Input: dimensioned drawing with shaded views. Units: mm. Origin: part minimum x, y, z. Round coordinates to 2 decimals unless told otherwise and drop trailing zeros. Order: outer loops, then holes, each group sorted by start corner. A loop starts at its lowest first (then second) coordinate and runs counter-clockwise, first axis right, second up. Notation, with made-up numbers: (66.5, 7) - (91.5, 7) arc R19 cw to (91.5, 17) - close; hole circle Ø7 at (86.5, -4). An arc over 180 degrees is marked (long way). Put each result on its own line as item: value. Start each with the question number.
(1) Section B-B (z = 10). Output: boundary loops of the cut face in (x, y), and give its area (3 significant figures).
(2) Section C-C (y = 56.5). Output: boundary loops of the cut face in (x, z), and give its area (3 significant figures).
(3) Material intervals for L1, parallel to Y at x = 21, z = 25; L2, parallel to Y at x = 24.5, z = 5.5 (1 decimal); L3, parallel to X at y = 62.5, z = 31.5, sorted ascending. Write a range as [from, to].
(4) Section D-D (y = 7.5). Output: boundary loops of the cut face in (x, z), and give its area (3 significant figures).
(5) Section A-A (x = 11.5). Output: boundary loops of the cut face in (y, z), and give its area (3 significant figures).
(6) Pin query (flat end, axial travel): P1, Ø5, axis at x = 27.5, y = 57.5, coming from the +Z side; P2, Ø5, axis at x = 12, z = 41.5, coming from the -Y side; P3, Ø10, axis at x = 24.5, y = 27.5, coming from the +Z side; P4, Ø2, axis at y = 11.5, z = 18, coming from the +X side. Return the tip coordinate at first contact, or that it passes through.
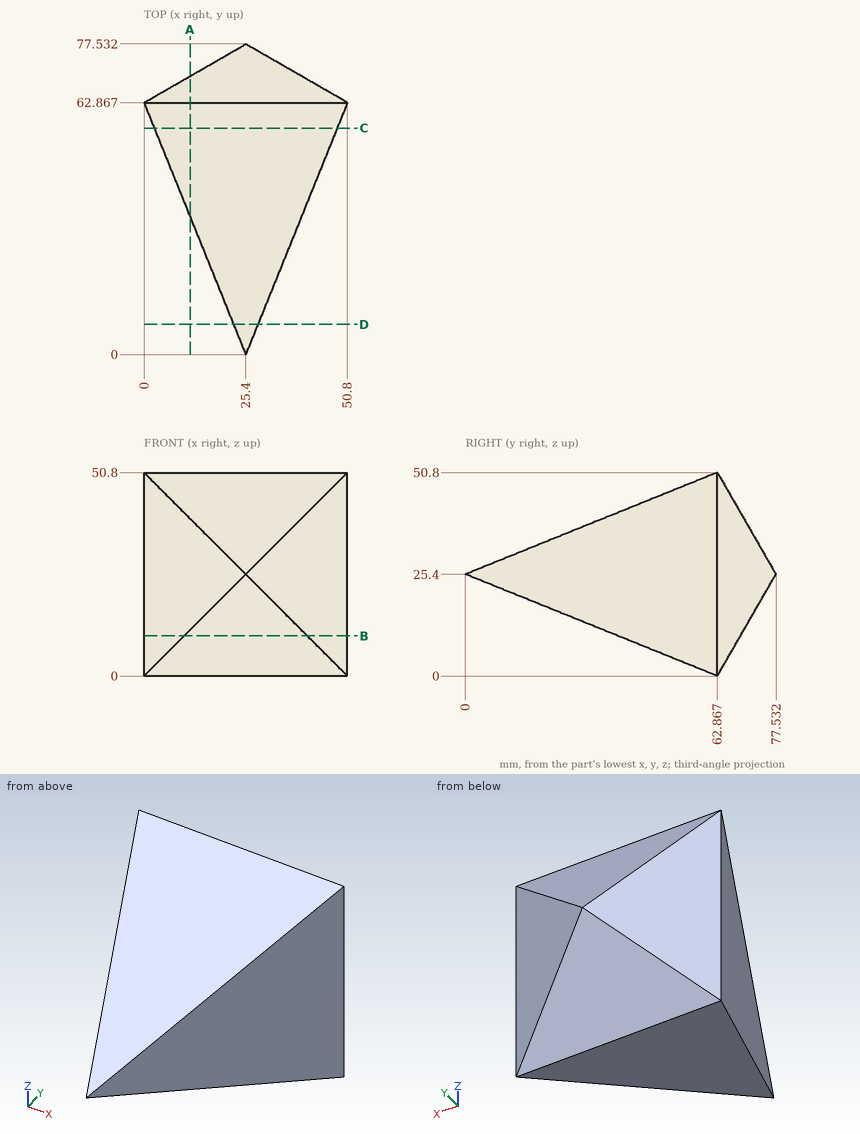
Checks:
1. outline: (0, 62.87) - (10, 38.12) - (40.8, 38.12) - (50.8, 62.87) - (40.8, 68.64) - (10, 68.64) - close
1. area: 1,250 mm²
2. outline: (2.57, 2.57) - (48.23, 2.57) - (48.23, 48.23) - (2.57, 48.23) - close
2. area: 2,080 mm²
3. L1: y = [10.89, 74.99]
3. L2: y = [49.3, 66]
3. L3: x = [0.15, 50.65]
4. outline: (22.37, 22.37) - (28.43, 22.37) - (28.43, 28.43) - (22.37, 28.43) - close
4. area: 36.7 mm²
5. outline: (34.4, 11.5) - (62.87, 0) - (69.51, 11.5) - (69.51, 39.3) - (62.87, 50.8) - (34.4, 39.3) - close
5. area: 1,380 mm²
6. P1: stops at z = 49.64
6. P2: stops at y = 33.66
6. P3: stops at z = 38.53
6. P4: passes through
